Read the model definition and answer for the solid it produces. Units are mm, in the model's axes. Face numbers are marked on the shaded views. Round coordinates to 2 decimals unless told otherwise and drop trailing zeros. Order: outer loops, then holes, each group sorted by start corner. A loop starts at its lowest first (then second) coordinate and runs counter-clockwise, first axis right, second up. Notation, with made-up numbers: (37, 64.25) -> (92, 64.25) arc R28 cw to (92, 100.25) -> close; hole circle Ø10 at (-30, 27.25). An arc over 180 degrees is marked (long way). One line per item, written item: value. Start each with the question number.
1. Section B-B (y = -93) is taken. Give the vertices of the cut face in (x, z).
2. Consider line 1 (Y direction, x = 32.5, z = -19); line 2 (X direction, y = -194.5, z = 5.5); line 3 (Z direction, x = 35.5, y = -641). Determine where each line is inside the solid, lowest interval first.
3. Section A-A (z = -12.5) is taken. Give the vertices of the cut face in (x, y).
4. The mould has two halves that part along Y. Classify the marked faces 1, 2 and 3: released by +Y, released by -Y, zero draft, split by the parting line, or undercut.
5. Section C-C (x = 52.5) is taken. Give the vertices of the cut face in (y, z).
6. Flat-ended cylindrical pins translate along their axes: pin 1 Ø8 at (x, y) = (2.5, -894.5) entering from +Z; pin 2 Ø16 at (x, z) = (-3.5, -8.5) entering from +Y. Find the tip coordinate at first contact, or state that the pin passes through.
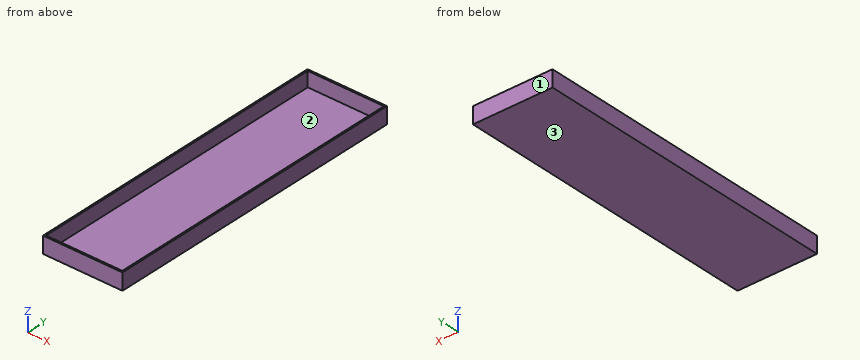
from build123d import *

# Parameters (mm, degrees)
F0_W     = 284
F0_H     = 59
F1_DEPTH = 1100
F3_DEPTH = 59
F4_W     = 272
F4_H     = 1088
F5_DEPTH = 53


with BuildPart() as f1:
    # F0 (on Front) → F1 (new body)
    with BuildSketch(Plane.XZ):
        Rectangle(F0_W, F0_H)
    extrude(amount=F1_DEPTH)

    # F2 (on face) → F3 (cut)
    with BuildSketch(Plane.XY.offset(29.5)):
        Polygon((148, 6), (-136, 6), (-136, 0), (142, 0), (142, -1094), (148, -1094), align=None)
    extrude(amount=-F3_DEPTH, mode=Mode.SUBTRACT)

    # F4 (on face) → F5 (cut)
    with BuildSketch(Plane.XY.offset(29.5)):
        with Locations((0, -550)):
            Rectangle(F4_W, F4_H)
    extrude(amount=-F5_DEPTH, mode=Mode.SUBTRACT)


solid = f1.part
Answer:
1. outline: (-142, -29.5) -> (142, -29.5) -> (142, 29.5) -> (136, 29.5) -> (136, -23.5) -> (-136, -23.5) -> (-136, 29.5) -> (-142, 29.5) -> close
2. line 1: -1100 to -1094, -6 to 0
2. line 2: -142 to -136, 136 to 142
2. line 3: -29.5 to -23.5
3. outline: (-142, -1100) -> (142, -1100) -> (142, 0) -> (-142, 0) -> close; hole (-136, -1094) -> (136, -1094) -> (136, -6) -> (-136, -6) -> close
4. face 1: released by +Y
4. face 2: undercut
4. face 3: zero draft
5. outline: (-1100, -29.5) -> (0, -29.5) -> (0, 29.5) -> (-6, 29.5) -> (-6, -23.5) -> (-1094, -23.5) -> (-1094, 29.5) -> (-1100, 29.5) -> close
6. pin 1: z = -23.5
6. pin 2: y = 0
